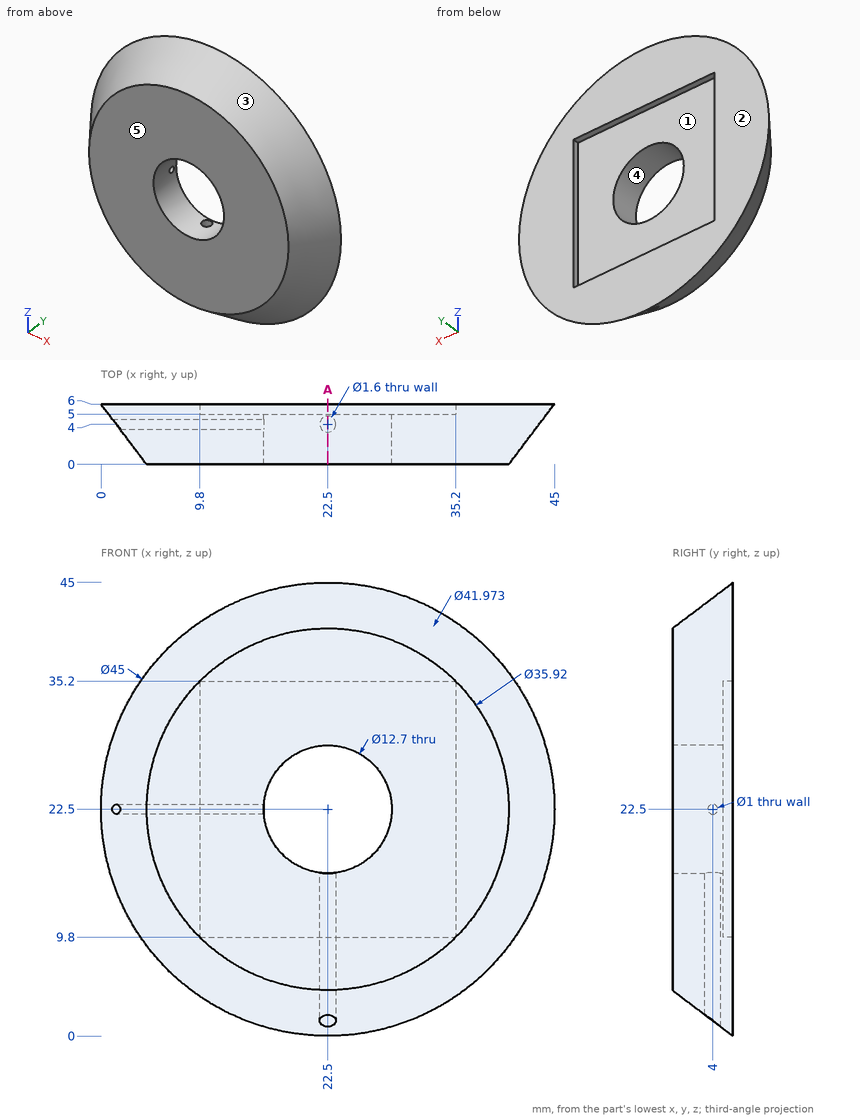
Check sheet for the drawn part. Datum: minimum x, y, z corner. Units: mm. A direction names the side the tool comes from. Give positions to 0.01 mm unless a question says otherwise; leave off trailing zeros. Write each loop counter-clockwise with the first axis right and the second up, starting at its lowest first coordinate (ties: lowest second). Pieces come first, ordered by that corner, then holes. Notation, with made-up numbers: M 40,-30.5 L 80,-30.5 A32 ccw 80,-2.5 Z; hole C 75,31.5 d2. An arc over 180 degrees is marked long. One line per question, with ' | ' between items.
1) Gauge pin test, flat ends, axial feed: pin 1 Ø3 at (x, y) = (16, 3.5) entering from +Z; pin 2 Ø1.8 at (x, y) = (22.5, 4) entering from -Z; pin 3 Ø5 at (x, z) = (29.5, 14) entering from +Y. Record the tip position at first contact, or that the pin passes through.
Result:
pin 1: stops at z = 43.33 | pin 2: stops at z = 0.83 | pin 3: stops at y = 5
2) Thickness scan on line 1 along Y through (x, z) = (31, 33.5); line 2 along Z through (x, y) = (4.5, 4.25) (1 decimal); line 3 along Y through (x, z) = (22, 5) (1 decimal). Record the ranges inside material, lowest first. Write a range as [from, to].
Result:
line 1: y = [0, 5] | line 2: z = [11.3, 22.1], [22.9, 33.7] | line 3: y = [0, 3.4], [4.6, 6]
3) Mould release check, pull along Z, two halves, no side actions. Record for the marked faces 3, 4 and 5: released by +Z, released by -Z, zero draft, split by the parting line, or undercut.
Result:
face 3: split by the parting line | face 4: undercut | face 5: zero draft
4) Section check A-A on x = 22.5. Enter the section's corners in (y, z).
Result:
outline: M 0,4.54 L 3.2,2.12 L 3.2,16.15 L 0,16.15 Z; M 0,28.85 L 5,28.85 L 5,35.2 L 6,35.2 L 6,45 L 0,40.46 Z; M 4.8,0.91 L 6,0 L 6,9.8 L 5,9.8 L 5,16.15 L 4.8,16.15 Z
5) Set-up check for the marked faces 1 and 2: record each of +Z, -Z, +X, -X, +Y, -Y from which the full face is reachable in a straight line by a thin tool's end or side.
Result:
face 1: +Y | face 2: +Z, -Z, +X, -X, +Y
